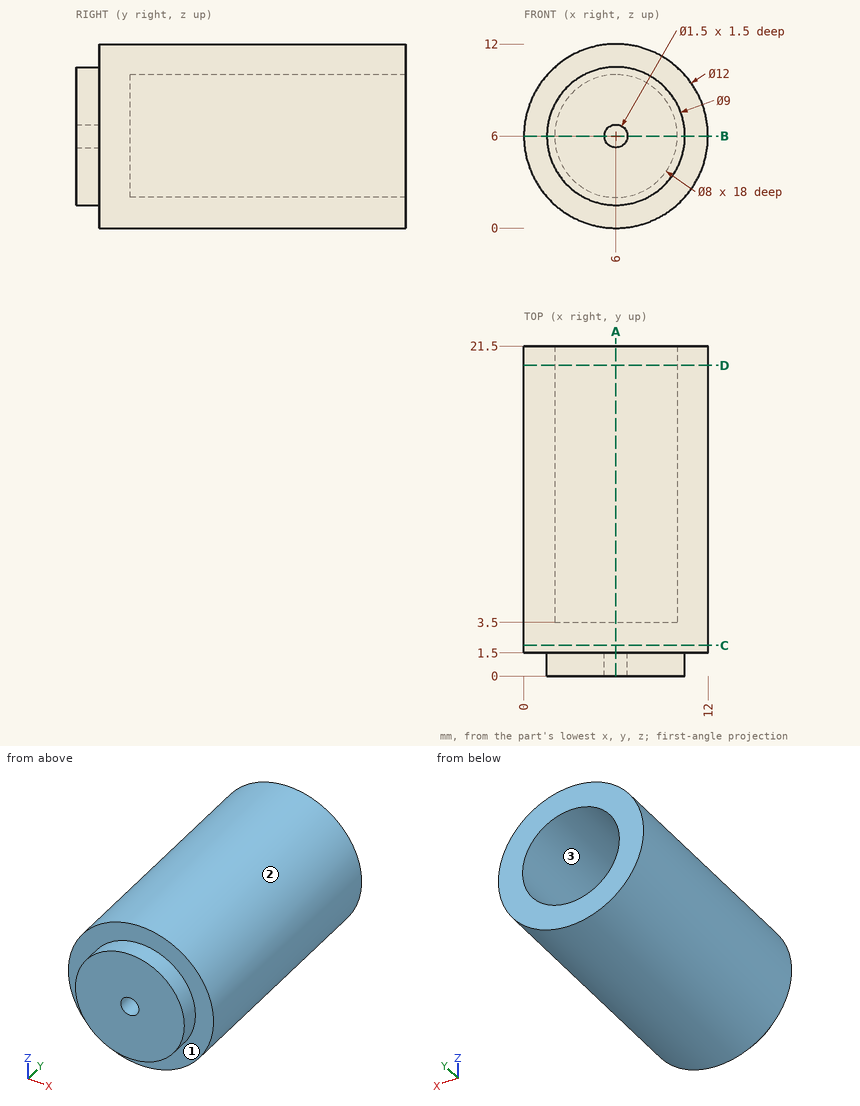
Geometry: see drawing. Coordinates: mm, zero at the bounding-box minimum. Round coordinates to 2 decimals unless told otherwise and drop trailing zeros. Loops run counter-clockwise (first coordinate to the right, second up) from the corner with the lowest first, then second, coordinate; pieces in that order, holes last. Notation, with made-up numbers: M -3.5,-17.5 L 9.5,-17.5 A15 ccw 9.5,8.5 Z; hole C 75.5,89 d6. An arc over 180 degrees is marked long. Use a Markdown table: item, result. Add a question column.
1. Ray query, line 1 along Z through (x, y) = (6, 0.35); line 2 along Z through (x, y) = (6, 8.25); line 3 along Y through (x, z) = (5, 7.25). Return the intervals inside material, ascending. Write a range as [from, to].
2. Contact query for flat-ended pins moving along their axis: pin 1 (5 mm diameter, centred on x = 2, y = 3.5, fed in from +Z); pin 2 (3 mm diameter, centred on y = 16, z = 9, fed in from -X); pin 3 (6 mm diameter, centred on y = 3.5, z = 2, fed in from -X). Output: stop coordinate, or through.
3. Cut plane A-A, the plane x = 6. Output: boundary loops of the cut face in (y, z), and give its area (3 significant figures).
4. Cut plane C-C, the plane y = 2. Output: boundary loops of the cut face in (x, z).
5. Cut plane B-B, the plane z = 6. Output: boundary loops of the cut face in (x, y), and give its area (3 significant figures).
6. Pull-direction query (X, two-part tool) for the marked faces 1, 2 and 3; classes: +X half, -X half, draft (parallel to the pull), parting line (faces both ways), or undercut.
7. Cut plane D-D, the plane y = 20.25. Output: boundary loops of the cut face in (x, z).
Solution:
| question | item | result |
|---|---|---|
| 1 | line 1 | z = [1.5, 5.25], [6.75, 10.5] |
| 1 | line 2 | z = [0, 2], [10, 12] |
| 1 | line 3 | y = [0, 3.5] |
| 2 | pin 1 | stops at z = 11.81 |
| 2 | pin 2 | stops at x = 0.19 |
| 2 | pin 3 | stops at x = 0.08 |
| 3 | outline | M 0,1.5 L 1.5,1.5 L 1.5,0 L 21.5,0 L 21.5,2 L 3.5,2 L 3.5,10 L 21.5,10 L 21.5,12 L 1.5,12 L 1.5,10.5 L 0,10.5 L 0,6.75 L 1.5,6.75 L 1.5,5.25 L 0,5.25 Z |
| 3 | area | 107 mm2 |
| 4 | outline | C 6,6 d12 |
| 5 | outline | M 0,1.5 L 1.5,1.5 L 1.5,0 L 5.25,0 L 5.25,1.5 L 6.75,1.5 L 6.75,0 L 10.5,0 L 10.5,1.5 L 12,1.5 L 12,21.5 L 10,21.5 L 10,3.5 L 2,3.5 L 2,21.5 L 0,21.5 Z |
| 5 | area | 107 mm2 |
| 6 | face 1 | draft |
| 6 | face 2 | parting line |
| 6 | face 3 | undercut |
| 7 | outline | C 6,6 d12; hole C 6,6 d8 |
